```python
from build123d import *

# Parameters (mm, degrees)
SKETCH_2_W               = 1.5
SKETCH_2_H               = 1.2
CUT_EXTRUDE_1_DEPTH      = 4
CUT_EXTRUDE_1_DEPTH_BACK = 4
CHAMFER_1_SIZE           = 0.4
FILLET_1_R               = 1
FILLET_2_R               = 0.4


with BuildPart() as part:
    # Эскиз1 → Повернуть1 (revolve)
    with BuildSketch(Plane(origin=(0, 0, 0), x_dir=(1, 0, 0), z_dir=(0, 1, 0))):
        Polygon((0, 0), (-3, 0), (-3, 1.8), (-1.5, 1.8), (-1.5, 11), (0, 11), align=None)
    revolve(axis=Axis((0, 0, -11), (0, 0, 1)))

    # Эскиз2 → Вырез-Вытянуть1 (cut, two sides)
    with BuildSketch(Plane(origin=(0, 0, 0), x_dir=(0, 0, -1), z_dir=(1, 0, 0))) as cut_extrude_1_sk:
        with Locations((0.75, 0)):
            Rectangle(SKETCH_2_W, SKETCH_2_H)
    extrude(amount=CUT_EXTRUDE_1_DEPTH, mode=Mode.SUBTRACT)
    extrude(cut_extrude_1_sk.sketch, amount=-CUT_EXTRUDE_1_DEPTH_BACK, mode=Mode.SUBTRACT)

    # Фаска1
    chamfer_1_edges = [part.edges().sort_by_distance(p)[0] for p in [
        (1.5, 0, -11),
    ]]
    chamfer(chamfer_1_edges, length=CHAMFER_1_SIZE)

    # Скругление1
    fillet_1_edges = [part.edges().sort_by_distance(p)[0] for p in [
        (0, 3, 0),
        (0, -3, 0),
    ]]
    fillet(fillet_1_edges, radius=FILLET_1_R)

    # Скругление2
    fillet_2_edges = [part.edges().sort_by_distance(p)[0] for p in [
        (1.5, 0, -1.8),
    ]]
    fillet(fillet_2_edges, radius=FILLET_2_R)


solid = part.part
```
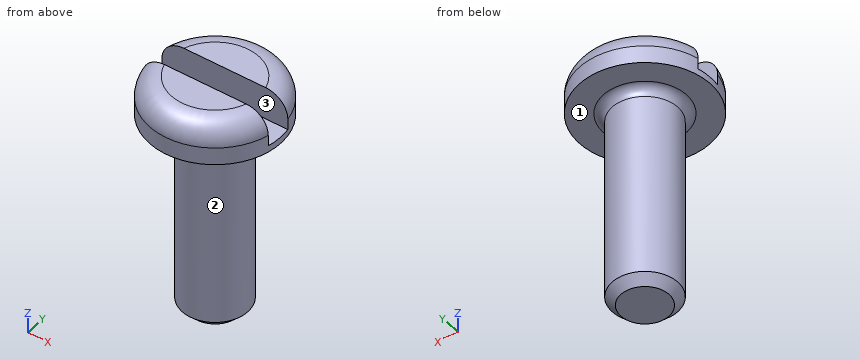
Read the model definition and answer for the solid it produces. Units are mm, in the model's axes. Face numbers are marked on the shaded views. Give positions to 0.01 mm unless a question says otherwise; leave off trailing zeros. Order: outer loops, then holes, each group sorted by start corner. A loop starts at its lowest first (then second) coordinate and runs counter-clockwise, first axis right, second up. Notation, with made-up numbers: (46.5, 28.25) -> (104.5, 28.25) arc R14 cw to (104.5, 36.25) -> close; hole circle Ø4 at (3, 0). An arc over 180 degrees is marked (long way). One line per item, written item: value. Start each with the question number.
(1) The part is cut by section B-B (x = 0). Determine the outline of the cut face in (y, z).
(2) Straight lines are drawn through the part: L1, parallel to Y at x = 0, z = -4; L2, parallel to Y at x = -2.6, z = -0.75. For each, find the intervals that lie inside material, in ascending order.
(3) For a pull along Y with two mould halves and no side action, classify the marked faces 1, 2 and 3 as released by +Y, released by -Y, zero draft, split by the parting line, or undercut.
(4) Flat-ended cylindrical pins translate along their axes: P1, Ø1.5, axis at y = 1, z = -3.5, coming from the +X side; P2, Ø0.8, axis at x = 1, z = -0.5, coming from the -Y side. Find the tip coordinate at first contact, or state that the pin passes through.
(5) The part is cut by section A-A (y = 0). Determine the outline of the cut face in (x, z).
(6) The part is cut by section C-C (z = -6). Determine the outline of the cut face in (x, y).
Taken from the geometry:
1. outline: (-3, -1.8) -> (-1.9, -1.8) arc R0.4 cw to (-1.5, -2.2) -> (-1.5, -10.6) -> (-1.1, -11) -> (1.1, -11) -> (1.5, -10.6) -> (1.5, -2.2) arc R0.4 cw to (1.9, -1.8) -> (3, -1.8) -> (3, -1) arc R1 ccw to (2, 0) -> (0.6, 0) -> (0.6, -1.5) -> (-0.6, -1.5) -> (-0.6, 0) -> (-2, 0) arc R1 ccw to (-3, -1) -> close
2. L1: -1.5 to 1.5
2. L2: -1.43 to -0.6, 0.6 to 1.43
3. face 1: zero draft
3. face 2: split by the parting line
3. face 3: undercut
4. P1: x = 1.48
4. P2: y = -2.89
5. outline: (-3, -1.8) -> (-1.9, -1.8) arc R0.4 cw to (-1.5, -2.2) -> (-1.5, -10.6) -> (-1.1, -11) -> (1.1, -11) -> (1.5, -10.6) -> (1.5, -2.2) arc R0.4 cw to (1.9, -1.8) -> (3, -1.8) -> (3, -1.5) -> (-3, -1.5) -> close
6. outline: circle Ø3 at (0, 0)
